```python
from build123d import *

# Parameters (mm, degrees)
F0_R     = 11
F1_DEPTH = 7
F3_DEPTH = 25


with BuildPart() as f1:
    # F0 (on Top) → F1 (new body)
    with BuildSketch(Plane.XY):
        with BuildLine():
            ThreePointArc((13.329884, 35.878532), (-12.10717, 37.855305), (-2.516762, 14.212644))
            ThreePointArc((-2.516762, 14.212644), (-22.596858, 8.130298), (-37.736662, -6.395248))
            ThreePointArc((-37.736662, -6.395248), (-26.73007, -29.41277), (-11.050129, -9.285902))
            ThreePointArc((-11.050129, -9.285902), (4.257384, -23.634602), (24.406778, -29.483284))
            ThreePointArc((24.406778, -29.483284), (38.837241, -8.442535), (13.566892, -4.926742))
            ThreePointArc((13.566892, -4.926742), (18.339474, 15.504304), (13.329884, 35.878532))
        make_face()
        with Locations((-25.114737, -14.5)):
            Circle(F0_R, mode=Mode.SUBTRACT)
        with Locations((25.114737, -14.5)):
            Circle(F0_R, mode=Mode.SUBTRACT)
        Circle(F0_R, mode=Mode.SUBTRACT)
        with Locations((0, 29)):
            Circle(F0_R, mode=Mode.SUBTRACT)
    extrude(amount=F1_DEPTH)

    # F2 (on face) → F3 (cut)
    with BuildSketch(Plane.XY.offset(7)):
        with BuildLine():
            ThreePointArc((13.643858, 22.767414), (9.670257, 17.53326), (3.840573, 14.5))
            ThreePointArc((3.840573, 14.5), (9.482877, 11.622179), (13.434387, 6.672125))
            ThreePointArc((13.434387, 6.672125), (14.336761, 14.709389), (13.643858, 22.767414))
        make_face()
        with BuildLine():
            ThreePointArc((-14.477655, -3.923966), (-14.806541, 2.401323), (-12.495423, 8.298458))
            ThreePointArc((-12.495423, 8.298458), (-19.907085, 5.061305), (-26.539088, 0.432221))
            ThreePointArc((-26.539088, 0.432221), (-20.019377, -0.391942), (-14.477655, -3.923966))
        make_face()
        with BuildLine():
            ThreePointArc((10.637082, -10.576034), (5.323663, -14.023502), (-0.938964, -14.970583))
            ThreePointArc((-0.938964, -14.970583), (5.570324, -19.770693), (12.89523, -23.199635))
            ThreePointArc((12.89523, -23.199635), (10.34912, -17.141318), (10.637082, -10.576034))
        make_face()
    extrude(amount=-F3_DEPTH, mode=Mode.SUBTRACT)


solid = f1.part
```
Input: part model. Units: mm. Frame: model coordinates. Coordinates: 2 decimals unless noted, no trailing zeros. Order: outer loops, then holes, each group sorted by start corner. A loop starts at its lowest first (then second) coordinate and runs counter-clockwise, first axis right, second up. Notation, with made-up numbers: (37, 66) - (57, 66) arc R13 cw to (57, 87) - close; hole circle Ø6 at (51.25, 33.25). An arc over 180 degrees is marked (long way). Return JSON: item names as keys, results as strings.
Q1. Draft query along X for faces 1 (the cylindrical face through (-33.844, -21.193, 3.451)), 2 (the flat face through (9, 7, 7)), 3 (the cylindrical face through (-2.38, -10.74, 3.45)). Return one class per face: +X half, -X half, draft (parallel to the pull), parting line (faces both ways), or undercut.
The answers:
{"face 1": "undercut", "face 2": "draft", "face 3": "undercut"}
Q2. Cut plane D-D (y = 29). Return loops of the section in (x, z), then the cut area to 3 significant figures.
The answers:
{"outline": "(-15, 0) - (-11, 0) - (-11, 7) - (-15, 7) - close; (11, 0) - (16.19, 0) - (16.19, 7) - (11, 7) - close", "area": "64.3 mm2"}
Q3. First-contact query: pin 1 (8 mm diameter, centred on x = 1.5, y = 23.5, fed in from +Z); pin 2 (3 mm diameter, centred on x = -1, z = 6, fed in from +Y); pin 3 (3 mm diameter, centred on y = 8.5, z = 3.5, fed in from -X). Flat tips, straight axial feed; report the tip coordinate or a pass-through.
The answers:
{"pin 1": "passes through", "pin 2": "stops at y = 44", "pin 3": "stops at x = -24.43"}
Q4. Cut plane A-A (x = 0). Return loops of the section in (y, z).
The answers:
{"outline": "(-20.88, 0) - (-15.79, 0) - (-15.79, 7) - (-20.88, 7) - close; (-15, 0) - (-11, 0) - (-11, 7) - (-15, 7) - close; (11, 0) - (18, 0) - (18, 7) - (11, 7) - close; (40, 0) - (44, 0) - (44, 7) - (40, 7) - close"}
Q5. Ray query, probe 1 along X at (y, z) = (-15.5, 0.5); probe 2 along X at (y, z) = (-8.5, 6.75); probe 3 along Y at (x, z) = (-13.5, 4.5). Return the intervals inside material, ascending.
The answers:
{"probe 1": "x = -40.08 to -36.07, -14.16 to -10.15, -6.12 to -0.34, 10.15 to 14.16, 36.07 to 40.08", "probe 2": "x = -38.86 to -34.33, -15.9 to -6.98, 6.98 to 15.9, 34.33 to 38.86", "probe 3": "y = -23.99 to 6.54, 7.96 to 12.18, 22.46 to 35.54"}
Q6. Cut plane B-B (z = 1.25). Return loops of the section in (x, y), then the cut area to 3 significant figures.
The answers:
{"outline": "(-37.74, -6.4) arc R15 ccw (long way) to (-11.05, -9.29) arc R45 ccw to (24.41, -29.48) arc R15 ccw (long way) to (13.57, -4.93) arc R45 ccw to (13.33, 35.88) arc R15 ccw (long way) to (-2.52, 14.21) arc R45 ccw to start; hole circle Ø22 at (-25.11, -14.5); hole (-26.54, 0.43) arc R15 cw to (-14.48, -3.92) arc R15 cw to (-12.5, 8.3) arc R41 ccw to start; hole circle Ø22 at (0, 0); hole circle Ø22 at (0, 29); hole (-0.94, -14.97) arc R41 ccw to (12.9, -23.2) arc R15 cw to (10.64, -10.58) arc R15 cw to start; hole (3.84, 14.5) arc R15 cw to (13.43, 6.67) arc R41 ccw to (13.64, 22.77) arc R15 cw to start; hole circle Ø22 at (25.11, -14.5)", "area": "1,580 mm2"}
Q7. Cut plane C-C (y = 2). Return loops of the section in (x, z).
The answers:
{"outline": "(-30.78, 0) - (-24.59, 0) - (-24.59, 7) - (-30.78, 7) - close; (-14.87, 0) - (-10.82, 0) - (-10.82, 7) - (-14.87, 7) - close; (10.82, 0) - (16.35, 0) - (16.35, 7) - (10.82, 7) - close"}
